Check sheet for the drawn part. Datum: minimum x, y, z corner. Units: mm. Round coordinates to 2 decimals unless told otherwise and drop trailing zeros. Loops run counter-clockwise (first coordinate to the right, second up) from the corner with the lowest first, then second, coordinate; pieces in that order, holes last. Notation, with made-up numbers: (46, 17.25) -> (82, 17.25) arc R29 cw to (82, 50.25) -> close; hole circle Ø4 at (-38, 12.5). An arc over 180 degrees is marked (long way). Write item = value, one per line. Start each with the question number.
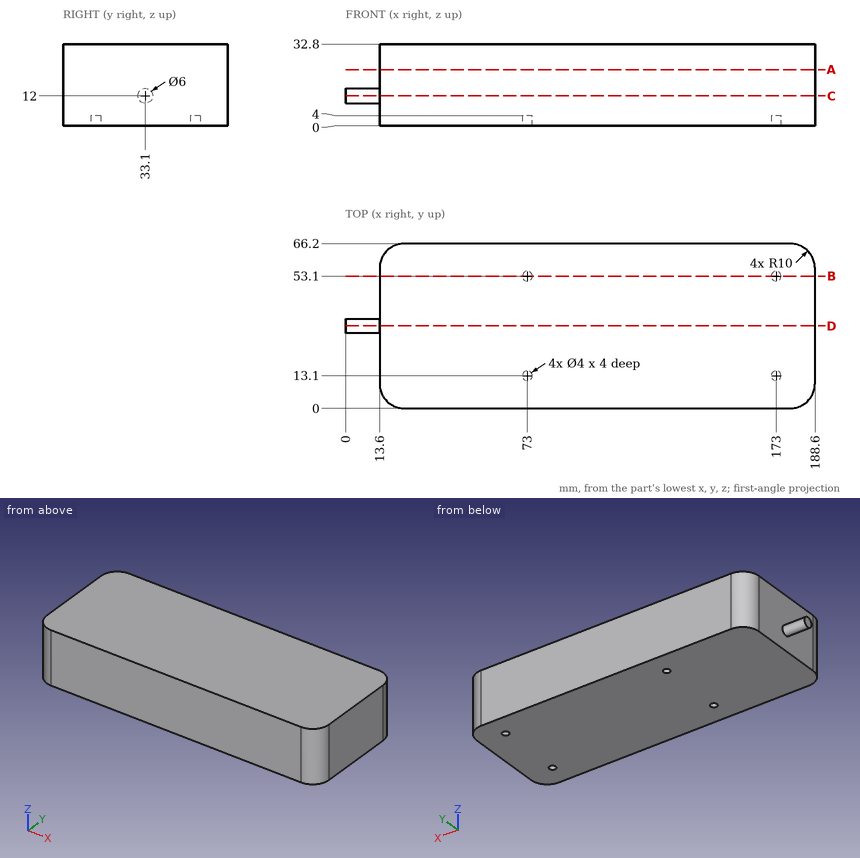
(1) Scan lines: line 1 (X direction, y = 53, z = 1); line 2 (Y direction, x = 173, z = 3); line 3 (X direction, y = 56, z = 19.5). Record each from-to range of solid material in increasing order. Write a range as [from, to].
(2) Section check B-B on y = 53.1. Enter the section's corners in (x, z), then the cut area to 3 significant figures.
(3) Depth check by flat-ended pin: pin 1 Ø10 at (y, z) = (28, 8.5) entering from -X; pin 2 Ø3.5 at (x, y) = (173, 13.1) entering from -Z; pin 3 Ø6 at (y, z) = (24, 13) entering from -X. Enter the tip coordinate at first touch or a pass-through.
(4) Section check A-A on z = 22.5. Enter the section's corners in (x, y).
(5) Section check C-C on z = 12. Enter the section's corners in (x, y).
(6) Section check D-D on y = 33.1. Enter the section's corners in (x, z).
Computed values:
q1.line_1 = [13.6, 71], [75, 171], [175, 188.6]
q1.line_2 = [0, 11.1], [15.1, 51.1], [55.1, 66.2]
q1.line_3 = [13.6, 188.6]
q2.outline = (13.6, 0) -> (71, 0) -> (71, 4) -> (75, 4) -> (75, 0) -> (171, 0) -> (171, 4) -> (175, 4) -> (175, 0) -> (188.6, 0) -> (188.6, 32.8) -> (13.6, 32.8) -> close
q2.area = 5,710 mm²
q3.pin_1 = 0
q3.pin_2 = 4
q3.pin_3 = 13.6
q4.outline = (13.6, 10) arc R10 ccw to (23.6, 0) -> (178.6, 0) arc R10 ccw to (188.6, 10) -> (188.6, 56.2) arc R10 ccw to (178.6, 66.2) -> (23.6, 66.2) arc R10 ccw to (13.6, 56.2) -> close
q5.outline = (0, 30.1) -> (13.6, 30.1) -> (13.6, 10) arc R10 ccw to (23.6, 0) -> (178.6, 0) arc R10 ccw to (188.6, 10) -> (188.6, 56.2) arc R10 ccw to (178.6, 66.2) -> (23.6, 66.2) arc R10 ccw to (13.6, 56.2) -> (13.6, 36.1) -> (0, 36.1) -> close
q6.outline = (0, 9) -> (13.6, 9) -> (13.6, 0) -> (188.6, 0) -> (188.6, 32.8) -> (13.6, 32.8) -> (13.6, 15) -> (0, 15) -> close
